The figure shows three views and two pictorial views of one solid part (mm, origin at its lowest corner). Answer the questions. A direction names the side the tool comes from. Give positions to 0.01 mm unless a question says otherwise; leave off trailing zeros. Order: outer loops, then holes, each group sorted by start corner. A loop starts at its lowest first (then second) coordinate and runs counter-clockwise, first axis right, second up. Notation, with made-up numbers: (51, -2) - (79, -2) arc R16 cw to (79, 26) - close; hole circle Ø2 at (45.5, 50.25). An arc over 180 degrees is marked (long way). Use a Markdown table: item, result. Add a question column.
1. A cutting plane is placed at A-A on y = 1.75. Determine the outline of the cut face in (x, z).
2. A cutting plane is placed at D-D on x = 38.1. Determine the outline of the cut face in (y, z), and give its area (3 significant figures).
3. Consider L1, parallel to X at y = 2.25, z = 10.5 (3 decimals); L2, parallel to Z at x = 29, y = 6; L3, parallel to X at y = 4.75, z = 60.5. Determine where each line is inside the solid, lowest interval first.
4. Which of the six approach directions +Z, -Z, +X, -X, +Y, -Y give full straight-line access (tool end or side, diameter ignored) to the marked faces 1, 2, 3, 4 and 5?
5. Flat-ended cylindrical pins translate along their axes: P1, Ø4.5, axis at y = 22, z = 39.5, coming from the -X side; P2, Ø8.5, axis at y = 5, z = 57, coming from the +X side; P3, Ø4, axis at x = 21.5, y = 5.5, coming from the +Z side. Find the tip coordinate at first contact, or state that the pin passes through.
6. A cutting plane is placed at C-C on z = 26.5. Determine the outline of the cut face in (x, y), and give its area (3 significant figures).
7. A cutting plane is placed at B-B on x = 54.5. Determine the outline of the cut face in (y, z).
8. For a pull along X with two mould halves and no side action, classify the marked faces 6, 7, 8 and 9 as released by +X, released by -X, zero draft, split by the parting line, or undercut.
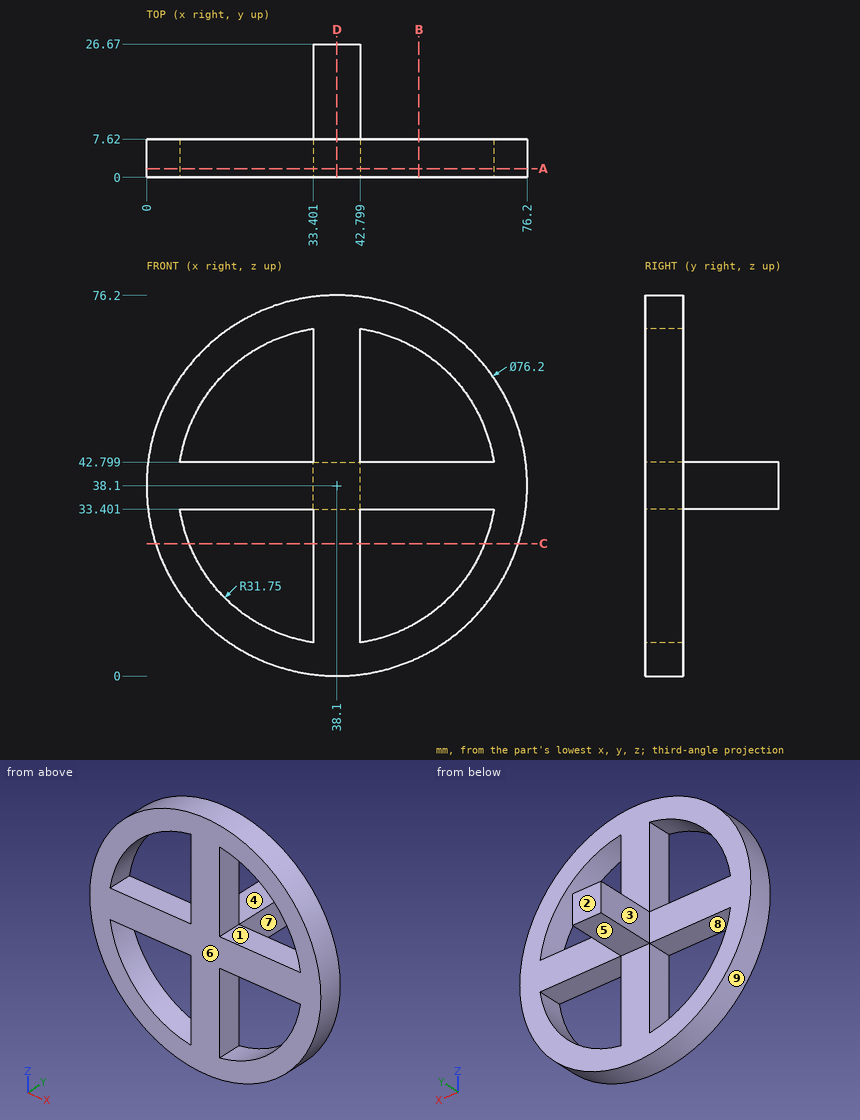
Output values:
| question | item | result |
|---|---|---|
| 1 | outline | circle Ø76.2 at (38.1, 38.1); hole (6.7, 33.4) arc R31.75 ccw to (33.4, 6.7) - (33.4, 33.4) - close; hole (6.7, 42.8) - (33.4, 42.8) - (33.4, 69.5) arc R31.75 ccw to start; hole (42.8, 6.7) arc R31.75 ccw to (69.5, 33.4) - (42.8, 33.4) - close; hole (42.8, 42.8) - (69.5, 42.8) arc R31.75 ccw to (42.8, 69.5) - close |
| 2 | outline | (0, 0) - (7.62, 0) - (7.62, 33.4) - (26.67, 33.4) - (26.67, 42.8) - (7.62, 42.8) - (7.62, 76.2) - (0, 76.2) - close |
| 2 | area | 760 mm² |
| 3 | L1 | 11.835 to 22.406, 33.401 to 42.799, 53.794 to 64.365 |
| 3 | L2 | 1.1 to 7.68, 33.4 to 42.8, 68.52 to 75.1 |
| 3 | L3 | 7.28 to 15.6, 33.4 to 42.8, 60.6 to 68.92 |
| 4 | face 1 | +Y, -Y |
| 4 | face 2 | +Z, -Z, +X, -X, +Y |
| 4 | face 3 | +Z, -Z, -X, +Y |
| 4 | face 4 | +Z, +X, -X, +Y |
| 4 | face 5 | -Z, +X, -X, +Y |
| 5 | P1 | x = 33.4 |
| 5 | P2 | x = 73.27 |
| 5 | P3 | z = 73.29 |
| 6 | outline | (1.81, 0) - (8.54, 0) - (8.54, 7.62) - (1.81, 7.62) - close; (33.4, 0) - (42.8, 0) - (42.8, 7.62) - (33.4, 7.62) - close; (67.66, 0) - (74.39, 0) - (74.39, 7.62) - (67.66, 7.62) - close |
| 6 | area | 174 mm² |
| 7 | outline | (0, 3.71) - (7.62, 3.71) - (7.62, 10.91) - (0, 10.91) - close; (0, 33.4) - (7.62, 33.4) - (7.62, 42.8) - (0, 42.8) - close; (0, 65.29) - (7.62, 65.29) - (7.62, 72.49) - (0, 72.49) - close |
| 8 | face 6 | zero draft |
| 8 | face 7 | released by +X |
| 8 | face 8 | undercut |
| 8 | face 9 | split by the parting line |
